from build123d import *

# Parameters (mm, degrees)
SKETCH1_W           = 59.69
SKETCH1_H           = 63.5
SKETCH1_R           = 2
BOSS_EXTRUDE1_DEPTH = 117
SKETCH2_W           = 50.165
SKETCH2_H           = 97.95
CUT_EXTRUDE1_DEPTH  = 138.033864953
SKETCH3_R           = 6
SKETCH3_R_2         = 3
CUT_EXTRUDE2_DEPTH  = 4.1
SKETCH5_R           = 3
CUT_EXTRUDE3_DEPTH  = 117.687481201


with BuildPart() as part:
    # Sketch1 → Boss-Extrude1 (new body)
    with BuildSketch(Plane.XY):
        with Locations((2.667, 0)):
            Rectangle(SKETCH1_W, SKETCH1_H)
        with Locations((-12.7, 0)):
            Circle(SKETCH1_R, mode=Mode.SUBTRACT)
        Circle(SKETCH1_R, mode=Mode.SUBTRACT)
        with Locations((12.7, 0)):
            Circle(SKETCH1_R, mode=Mode.SUBTRACT)
    extrude(amount=BOSS_EXTRUDE1_DEPTH)

    # Sketch2 → Cut-Extrude1 (cut, through all)
    with BuildSketch(Plane.XZ.offset(31.75)):
        with Locations((-2.0955, 58.5)):
            Rectangle(SKETCH2_W, SKETCH2_H)
    extrude(amount=-CUT_EXTRUDE1_DEPTH, mode=Mode.SUBTRACT)

    # Sketch3 → Cut-Extrude2 (cut)
    # profile 1 of 4: a face of its own
    with BuildSketch(Plane.XY.offset(9.525)):
        with Locations((-17.178, -21.75)):
            Circle(SKETCH3_R)
        with Locations((-17.178, -21.75)):
            Circle(SKETCH3_R_2, mode=Mode.SUBTRACT)
    # profile 2 of 4: a face of its own
    with BuildSketch(Plane.XY.offset(9.525)):
        with Locations((7.822, -21.75)):
            Circle(SKETCH3_R)
        with Locations((7.822, -21.75)):
            Circle(SKETCH3_R_2, mode=Mode.SUBTRACT)
    # profile 3 of 4: a face of its own
    with BuildSketch(Plane.XY.offset(9.525)):
        with Locations((-17.178, 21.75)):
            Circle(SKETCH3_R)
        with Locations((-17.178, 21.75)):
            Circle(SKETCH3_R_2, mode=Mode.SUBTRACT)
    # profile 4 of 4: a face of its own
    with BuildSketch(Plane.XY.offset(9.525)):
        with Locations((7.822, 21.75)):
            Circle(SKETCH3_R)
        with Locations((7.822, 21.75)):
            Circle(SKETCH3_R_2, mode=Mode.SUBTRACT)
    extrude(amount=-CUT_EXTRUDE2_DEPTH, mode=Mode.SUBTRACT)

    # Sketch5 → Cut-Extrude3 (cut, through all)
    with BuildSketch(Plane.XY.offset(9.525)):
        with Locations((-17.178, 21.75)):
            Circle(SKETCH5_R)
        with Locations((7.822, 21.75)):
            Circle(SKETCH5_R)
        with Locations((7.822, -21.75)):
            Circle(SKETCH5_R)
        with Locations((-17.178, -21.75)):
            Circle(SKETCH5_R)
    extrude(amount=-CUT_EXTRUDE3_DEPTH, mode=Mode.SUBTRACT)


solid = part.part
Source: CAD feature listing. Evaluate the final solid. Frame: model axes, mm. A direction names the side the tool comes from. Coordinates: 2 decimals unless noted, no trailing zeros. Loops run counter-clockwise (first coordinate to the right, second up) from the corner with the lowest first, then second, coordinate; pieces in that order, holes last. Notation, with made-up numbers: (-4.75, 54) -> (43.25, 54) arc R19 cw to (43.25, 81) -> close; hole circle Ø11 at (-32, 50.5). An arc over 180 degrees is marked (long way). Answer in a Markdown table with one row per item. Add a question column.
Q1. Contact query for flat-ended pins moving along their axis: pin 1 Ø3.5 at (x, y) = (12.7, 0) entering from -Z; pin 2 Ø12 at (y, z) = (-13.5, 81) entering from -X. Output: stop coordinate, or through.
Q2. Section A-A on x = 0. Return the cut outline in (y, z) (3 decimals), and give its area (3 significant figures).
Q3. Section D-D on y = 0. Give the number of separate pieces and of enclosed holes in the cut face, and give its area (3 significant figures).
Q4. Pull-direction query (Y, two-part tool) for faces 5 (the face through (-16, 25, 5.425)), 6 (the face through (25, -31.75, 58)), 7 (the face through (2.2, 0.4, 117)); classes: pulls with the +Y half, pulls with the -Y half, needs draft (parallel to the pull), parting line crosses it, or undercut.
Q5. Section C-C on x = -7. Return the cut outline in (y, z) (3 decimals).
Q6. Section B-B on y = -21.75. Return the cut outline in (x, z) (3 decimals).
Q7. Ray query, line 1 along X through (y, z) = (0, 6.75); line 2 along Z through (x, y) = (15, 22.5) (3 decimals); line 3 along Z through (x, y) = (-15.5, 25) (3 decimals). Return the intervals inside material, ascending.
Q8. Reachability of faces 1 (the face through (-2.4, -0.4, 107.475)), 2 (the face through (9.21, -24.41, 2.75)), 3 (the face through (1.828, -21.486, 7.504)), 4 (the face through (25, 31.75, 58)) from +Z, -Z, +X, -X, +Y, -Y: full face, straight path, thin tool, end or side. Return the list, or none.
Computed values:
| question | item | result |
|---|---|---|
| 1 | pin 1 | passes through |
| 1 | pin 2 | stops at x = 22.99 |
| 2 | outline | (-31.75, 0) -> (-2, 0) -> (-2, 9.525) -> (-31.75, 9.525) -> close; (-31.75, 107.475) -> (-2, 107.475) -> (-2, 117) -> (-31.75, 117) -> close; (2, 0) -> (31.75, 0) -> (31.75, 9.525) -> (2, 9.525) -> close; (2, 107.475) -> (31.75, 107.475) -> (31.75, 117) -> (2, 117) -> close |
| 2 | area | 1,130 mm^2 |
| 3 | separate pieces | 7 |
| 3 | enclosed holes | 0 |
| 3 | area | 1,840 mm^2 |
| 4 | face 5 | undercut |
| 4 | face 6 | pulls with the -Y half |
| 4 | face 7 | needs draft |
| 5 | outline | (-31.75, 0) -> (31.75, 0) -> (31.75, 9.525) -> (-31.75, 9.525) -> close; (-31.75, 107.475) -> (31.75, 107.475) -> (31.75, 117) -> (-31.75, 117) -> close |
| 6 | outline | (-27.178, 0) -> (-20.178, 0) -> (-20.178, 5.425) -> (-23.178, 5.425) -> (-23.178, 9.525) -> (-27.178, 9.525) -> close; (-27.178, 107.475) -> (22.987, 107.475) -> (22.987, 9.525) -> (13.822, 9.525) -> (13.822, 5.425) -> (10.822, 5.425) -> (10.822, 0) -> (32.512, 0) -> (32.512, 117) -> (-27.178, 117) -> close; (-14.178, 0) -> (4.822, 0) -> (4.822, 5.425) -> (1.822, 5.425) -> (1.822, 9.525) -> (-11.178, 9.525) -> (-11.178, 5.425) -> (-14.178, 5.425) -> close |
| 7 | line 1 | x = -27.18 to -14.7, -10.7 to -2, 2 to 10.7, 14.7 to 32.51 |
| 7 | line 2 | z = 0 to 9.525, 107.475 to 117 |
| 7 | line 3 | z = 0 to 5.425, 107.475 to 117 |
| 8 | face 1 | -X, +Y, -Y |
| 8 | face 2 | -Z |
| 8 | face 3 | none |
| 8 | face 4 | +Z, -Z, +X, -X, +Y |
